Source: three-view drawing plus pictorial views. Frame: mm from the lowest corner of the part. Round coordinates to 2 decimals unless told otherwise and drop trailing zeros. Write each loop counter-clockwise with the first axis right and the second up, starting at its lowest first coordinate (ties: lowest second). Pieces come first, ordered by that corner, then holes. Notation, with made-up numbers: M 55,-15.5 L 102,-15.5 A15 cw 102,-7.5 Z; hole C 29.5,47 d3. An arc over 180 degrees is marked long. Answer as CSV lines item,"result". Start each with the question number.
Q1. Section query A-A on z = 55. Output: boundary loops of the cut face in (x, y).
Q2. Section query B-B on z = 77.5. Give the number of separate pieces and of enclosed holes in the cut face, and give its area (3 significant figures).
Q3. First-contact query: pin 1 (1.5 mm diameter, centred on x = 65, y = 1.5, fed in from +Z). Flat tip, straight axial feed; report the tip coordinate or a pass-through.
Q4. Ray query, probe 1 along X at (y, z) = (1.7, 55); probe 2 along X at (y, z) = (0.7, 77.5); probe 3 along X at (y, z) = (1.8, 77.5). Return the intervals inside material, ascending.
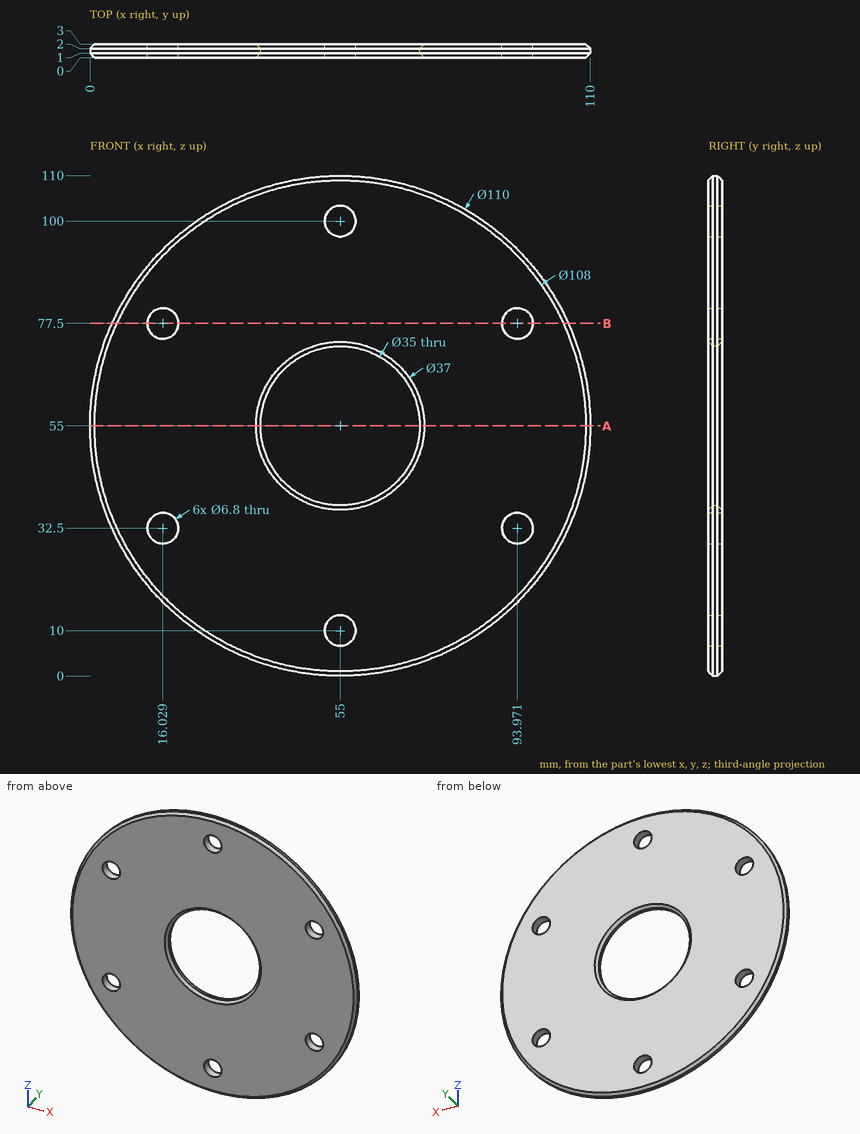
Entries:
1,outline,"M 0,1 L 1,0 L 36.5,0 L 37.5,1 L 37.5,2 L 36.5,3 L 1,3 L 0,2 Z; M 72.5,1 L 73.5,0 L 109,0 L 110,1 L 110,2 L 109,3 L 73.5,3 L 72.5,2 Z"
2,separate pieces,"3"
2,enclosed holes,"0"
2,area,"258 mm^2"
3,pin 1,"stops at z = 109.22"
4,probe 1,"x = 0 to 37.5, 72.5 to 110"
4,probe 2,"x = 5.14 to 12.63, 19.43 to 90.57, 97.37 to 104.86"
4,probe 3,"x = 4.81 to 12.63, 19.43 to 90.57, 97.37 to 105.19"
